from build123d import *

# Parameters (mm, degrees)
SKETCH_1_W             = 200
SKETCH_1_H             = 80
EXTRUDE_1_DEPTH        = 5
SKETCH_2_W             = 160
SKETCH_2_H             = 80
EXTRUDE_2_DEPTH        = 25
CUT_EXTRUDE_START      = -5
SKETCH_3_W             = 150
SKETCH_3_H             = 65
CUT_EXTRUDE_1_DEPTH    = 20
HOLE_WIZARD_M6_1_D     = 5
HOLE_WIZARD_M6_1_DEPTH = 15
HOLE_WIZARD_M6_1_TIP   = 1.502151548


with BuildPart() as part:
    # 草图1 → 凸台-拉伸1 (new body)
    with BuildSketch(Plane.XY):
        Rectangle(SKETCH_1_W, SKETCH_1_H)
    extrude(amount=EXTRUDE_1_DEPTH)

    # 草图2 → 凸台-拉伸2 (add)
    with BuildSketch(Plane.XY.offset(5)):
        Rectangle(SKETCH_2_W, SKETCH_2_H)
    extrude(amount=EXTRUDE_2_DEPTH)

    # 草图3 → 切除-拉伸1 (cut)
    with BuildSketch(Plane.XY.offset(30).offset(CUT_EXTRUDE_START)):
        Rectangle(SKETCH_3_W, SKETCH_3_H)
    extrude(amount=-CUT_EXTRUDE_1_DEPTH, mode=Mode.SUBTRACT)

    # M6 螺纹孔1
    with Locations(Plane.XY.offset(5)):
        with Locations((-90, 30), (-90, -30), (90, 30), (90, -30)):
            Hole(HOLE_WIZARD_M6_1_D / 2, depth=HOLE_WIZARD_M6_1_DEPTH)
            with Locations((0, 0, -(HOLE_WIZARD_M6_1_DEPTH + HOLE_WIZARD_M6_1_TIP / 2))):  # 118° drill point
                Cone(0, HOLE_WIZARD_M6_1_D / 2, HOLE_WIZARD_M6_1_TIP, mode=Mode.SUBTRACT)


solid = part.part
Work out the finished part from the listing and answer in its coordinate system (mm). A direction names the side the tool comes from. Give positions to 0.01 mm unless a question says otherwise; leave off trailing zeros. Loops run counter-clockwise (first coordinate to the right, second up) from the corner with the lowest first, then second, coordinate; pieces in that order, holes last. Notation, with made-up numbers: (-2, -10.75) -> (9, -10.75) arc R31 cw to (9, 15.25) -> close; hole circle Ø1 at (49, -7). An arc over 180 degrees is marked (long way). Use a Markdown table: item, result. Add a question column.
1. For faces 5 (the cylindrical face through (-88.16, 31.69, 2.46)), 6 (the flat face through (-1, 1, 0)), 7 (the flat face through (-1, 0, 5)), 8 (the flat face through (80, -1, 17)), 9 (the flat face through (-80, -1, 17)), determine the directions among +Z, -Z, +X, -X, +Y, -Y from which every point of the face is accessible in a straight line to the end or side of a thin tool.
2. Section B-B on x = -22.5 is taken. Determine the outline of the cut face in (y, z), and give its area (3 significant figures).
3. Flat-ended cylindrical pins translate along their axes: pin 1 Ø12 at (y, z) = (32, 13.5) entering from +X; pin 2 Ø1.5 at (y, z) = (19.5, 24.5) entering from -X; pin 3 Ø6 at (x, y) = (-91, 1) entering from +Z. Find the tip coordinate at first contact, or state that the pin passes through.
4. Determine the mould class of faces 1 (the flat face through (-1, -40, 15)), 2 (the flat face through (100, -1, 2)), 3 (the flat face through (-1, 0, 25)), 4 (the cylindrical face through (-88.16, -28.31, 2.46)) for opening direction X: released by +X, released by -X, zero draft, split by the parting line, or undercut.
5. Section D-D on z = 21.5 is taken. Determine the outline of the cut face in (x, y), and give its area (3 significant figures).
6. Section C-C on x = -90 is taken. Determine the outline of the cut face in (y, z), and give its area (3 significant figures).
7. Find the intervals of material crossed by probe 1 along Y at (x, z) = (90, 2.1); probe 2 along Z at (x, y) = (-27.5, -3); probe 3 along X at (y, z) = (-22, 17.75), in increasing order.
8. Section A-A on y = 30 is taken. Determine the outline of the cut face in (x, z).
Results below:
| question | item | result |
|---|---|---|
| 1 | face 5 | +Z, -Z |
| 1 | face 6 | -Z, +X, -X, +Y, -Y |
| 1 | face 7 | none |
| 1 | face 8 | +Z, +X, +Y, -Y |
| 1 | face 9 | +Z, -X, +Y, -Y |
| 2 | outline | (-40, 0) -> (40, 0) -> (40, 30) -> (-40, 30) -> close; hole (-32.5, 5) -> (32.5, 5) -> (32.5, 25) -> (-32.5, 25) -> close |
| 2 | area | 1,100 mm^2 |
| 3 | pin 1 | stops at x = 80 |
| 3 | pin 2 | stops at x = -80 |
| 3 | pin 3 | stops at z = 5 |
| 4 | face 1 | zero draft |
| 4 | face 2 | released by +X |
| 4 | face 3 | undercut |
| 4 | face 4 | undercut |
| 5 | outline | (-80, -40) -> (80, -40) -> (80, 40) -> (-80, 40) -> close; hole (-75, -32.5) -> (75, -32.5) -> (75, 32.5) -> (-75, 32.5) -> close |
| 5 | area | 3,050 mm^2 |
| 6 | outline | (-40, 0) -> (-32.5, 0) -> (-32.5, 5) -> (-40, 5) -> close; (-27.5, 0) -> (27.5, 0) -> (27.5, 5) -> (-27.5, 5) -> close; (32.5, 0) -> (40, 0) -> (40, 5) -> (32.5, 5) -> close |
| 6 | area | 350 mm^2 |
| 7 | probe 1 | y = -40 to -32.5, -27.5 to 27.5, 32.5 to 40 |
| 7 | probe 2 | z = 0 to 5, 25 to 30 |
| 7 | probe 3 | x = -80 to -75, 75 to 80 |
| 8 | outline | (-100, 0) -> (-92.5, 0) -> (-92.5, 5) -> (-100, 5) -> close; (-87.5, 0) -> (87.5, 0) -> (87.5, 5) -> (80, 5) -> (80, 30) -> (-80, 30) -> (-80, 5) -> (-87.5, 5) -> close; (92.5, 0) -> (100, 0) -> (100, 5) -> (92.5, 5) -> close; hole (-75, 5) -> (75, 5) -> (75, 25) -> (-75, 25) -> close |
